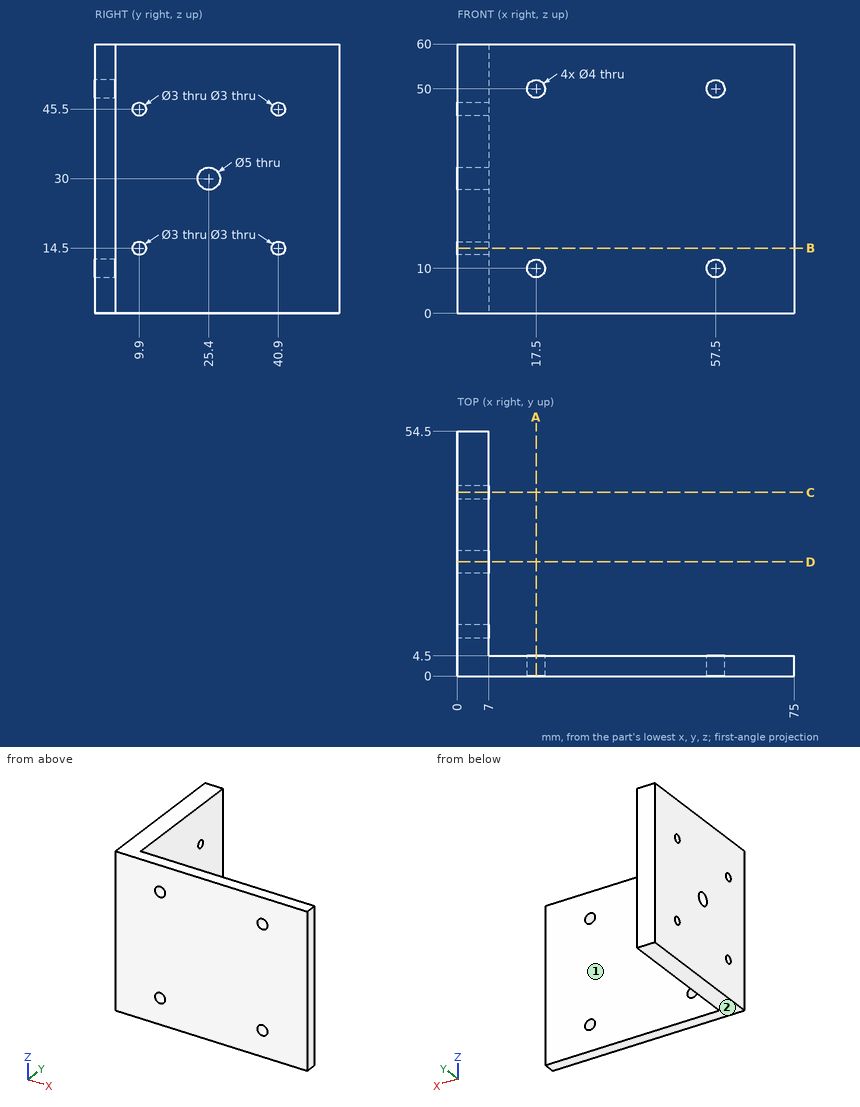
Geometry: see drawing. Coordinates: mm, zero at the bounding-box minimum. A direction names the side the tool comes from. Round coordinates to 2 decimals unless told otherwise and drop trailing zeros. Write each loop counter-clockwise with the first axis right and the second up, starting at its lowest first coordinate (ties: lowest second). Pieces come first, ordered by that corner, then holes.
1) Cut plane A-A (x = 17.5). Return the cut outline in (y, z), then the cut area to 3 significant figures.
2) Ray query, L1, parallel to X at y = 2.5, z = 10; L2, parallel to Y at x = 4.25, z = 30; L3, parallel to X at y = 16, z = 10. Return the intervals inside material, ascending.
3) Reachability of the marked faces 1 and 2 from +Z, -Z, +X, -X, +Y, -Y: full face, straight path, thin tool, end or side. Return the list, or none.
4) Contact query for flat-ended pins moving along their axis: P1, Ø5, axis at x = 36, z = 36, coming from the +Y side; P2, Ø6.5, axis at y = 25.4, z = 30, coming from the +X side; P3, Ø1.8, axis at y = 40.9, z = 45.5, coming from the +X side; P4, Ø4, axis at y = 34.5, z = 53.5, coming from the -X side. Output: stop coordinate, or through.
5) Cut plane B-B (z = 14.5). Return the cut outline in (x, y).
6) Cut plane D-D (y = 25.4). Return the cut outline in (x, z).
7) Cut plane C-C (y = 40.9). Return the cut outline in (x, z).
Geometry says:
1. outline: (0, 0) - (4.5, 0) - (4.5, 8) - (0, 8) - close; (0, 12) - (4.5, 12) - (4.5, 48) - (0, 48) - close; (0, 52) - (4.5, 52) - (4.5, 60) - (0, 60) - close
1. area: 234 mm2
2. L1: x = 0 to 15.5, 19.5 to 55.5, 59.5 to 75
2. L2: y = 0 to 22.9, 27.9 to 54.5
2. L3: x = 0 to 7
3. face 1: +Z, -Z, +X, +Y
3. face 2: -Z, +X, -X, +Y, -Y
4. P1: stops at y = 4.5
4. P2: stops at x = 7
4. P3: passes through
4. P4: stops at x = 0
5. outline: (0, 0) - (75, 0) - (75, 4.5) - (7, 4.5) - (7, 8.4) - (0, 8.4) - close; (0, 11.4) - (7, 11.4) - (7, 39.4) - (0, 39.4) - close; (0, 42.4) - (7, 42.4) - (7, 54.5) - (0, 54.5) - close
6. outline: (0, 0) - (7, 0) - (7, 27.5) - (0, 27.5) - close; (0, 32.5) - (7, 32.5) - (7, 60) - (0, 60) - close
7. outline: (0, 0) - (7, 0) - (7, 13) - (0, 13) - close; (0, 16) - (7, 16) - (7, 44) - (0, 44) - close; (0, 47) - (7, 47) - (7, 60) - (0, 60) - close
